Geometry check sheet. Reference: the model listing, model coordinates, mm. A direction names the side the tool comes from. Round coordinates to 2 decimals unless told otherwise and drop trailing zeros. Write each loop counter-clockwise with the first axis right and the second up, starting at its lowest first coordinate (ties: lowest second). Pieces come first, ordered by that corner, then holes. Notation, with made-up numbers: (-5, -31) -> (10, -31) arc R5 ccw to (10, -24) -> close; hole circle Ø5 at (69.25, -15). An arc over 180 degrees is marked (long way). Use a Markdown table: item, result.
```python
from build123d import *

# Parameters (mm, degrees)
BOSS_EXTRUDE1_DEPTH = 4
SKETCH2_R           = 20
BOSS_EXTRUDE2_DEPTH = 4
SKETCH3_R           = 20
BOSS_EXTRUDE3_DEPTH = 4
CUT_EXTRUDE2_DEPTH  = 8
FILLET1_R           = 3
FILLET2_R           = 1


with BuildPart() as part:
    # Sketch1 → Boss-Extrude1 (new, symmetric)
    with BuildSketch(Plane.XY):
        with BuildLine():
            Line((195, 89.5), (-195, 89.5))
            ThreePointArc((-195, 89.5), (-216.213203436, 80.713203436), (-225, 59.5))
            Line((-225, 59.5), (-225, -59.5))
            ThreePointArc((-225, -59.5), (-216.213203436, -80.713203436), (-195, -89.5))
            Line((-195, -89.5), (195, -89.5))
            ThreePointArc((195, -89.5), (216.213203436, -80.713203436), (225, -59.5))
            Line((225, -59.5), (225, 59.5))
            ThreePointArc((225, 59.5), (216.213203436, 80.713203436), (195, 89.5))
        make_face()
    extrude(amount=BOSS_EXTRUDE1_DEPTH, both=True)

    # Sketch2 → Boss-Extrude2 (add, symmetric)
    with BuildSketch(Plane.XY.offset(4)):
        with Locations(Location((-185, 0, 0), (0, 0, 180))):
            Circle(SKETCH2_R)
        with Locations(Location((185, 0, 0), (0, 0, 180))):
            Circle(SKETCH2_R)
    extrude(amount=BOSS_EXTRUDE2_DEPTH, both=True)

    # Sketch3 → Boss-Extrude3 (add, symmetric)
    with BuildSketch(Plane.XY.offset(4)):
        with Locations(Location((0, 0, 0), (0, 0, 180))):
            Circle(SKETCH3_R)
    extrude(amount=BOSS_EXTRUDE3_DEPTH, both=True)

    # Sketch4 → Cut-Extrude2 (cut)
    with BuildSketch(Plane.XY.offset(4)):
        with BuildLine():
            Line((-168.5, 59), (-131.5, 59))
            ThreePointArc((-131.5, 59), (-127.5, 55), (-131.5, 51))
            Line((-131.5, 51), (-168.5, 51))
            ThreePointArc((-168.5, 51), (-172.5, 55), (-168.5, 59))
        make_face()
        with BuildLine():
            Line((168.5, 59), (131.5, 59))
            ThreePointArc((131.5, 59), (127.5, 55), (131.5, 51))
            Line((131.5, 51), (168.5, 51))
            ThreePointArc((168.5, 51), (172.5, 55), (168.5, 59))
        make_face()
        with BuildLine():
            Line((-168.5, -59), (-131.5, -59))
            ThreePointArc((-131.5, -59), (-127.5, -55), (-131.5, -51))
            Line((-131.5, -51), (-168.5, -51))
            ThreePointArc((-168.5, -51), (-172.5, -55), (-168.5, -59))
        make_face()
        with BuildLine():
            Line((168.5, -59), (131.5, -59))
            ThreePointArc((131.5, -59), (127.5, -55), (131.5, -51))
            Line((131.5, -51), (168.5, -51))
            ThreePointArc((168.5, -51), (172.5, -55), (168.5, -59))
        make_face()
    extrude(amount=-CUT_EXTRUDE2_DEPTH, mode=Mode.SUBTRACT)

    # Fillet1
    fillet1_edges = [part.edges().sort_by_distance(p)[0] for p in [
        (225, 0, -4),
        (216.213203436, -80.713203436, -4),
        (0, -89.5, -4),
        (-216.213203436, -80.713203436, -4),
        (216.213203436, -80.713203436, 4),
        (225, 0, 4),
        (216.213203436, 80.713203436, 4),
        (0, 89.5, 4),
        (-216.213203436, 80.713203436, 4),
        (-225, 0, 4),
        (-216.213203436, -80.713203436, 4),
        (-225, 0, -4),
        (0, -89.5, 4),
        (-216.213203436, 80.713203436, -4),
        (0, 89.5, -4),
        (216.213203436, 80.713203436, -4),
    ]]
    fillet(fillet1_edges, radius=FILLET1_R)

    # Fillet2
    fillet2_edges = [part.edges().sort_by_distance(p)[0] for p in [
        (205, 0, 8),
        (-165, 0, 8),
        (20, 0, 8),
    ]]
    fillet(fillet2_edges, radius=FILLET2_R)


solid = part.part
```
(1) Gauge pin test, flat ends, axial feed: pin 1 Ø6 at (y, z) = (40, 1.5) entering from -X; pin 2 Ø3 at (y, z) = (-44.5, 3) entering from +X; pin 3 Ø5 at (y, z) = (-44, 5.5) entering from -X. Record the tip position at first contact, or that the pin passes through.
A:
| item | result |
|---|---|
| pin 1 | stops at x = -225 |
| pin 2 | stops at x = 224.96 |
| pin 3 | stops at x = -224.24 |
(2) Release check for a two-part mould opening along Y. For faces 4 (the face through (216.445, 80.479, 0.014)), 5 (the face through (-150, -59, 0)), 6 (the face through (172.5, 54.9, 0.1)), 7 (the face through (-216.445, -80.479, 0.014)) record: +Y half, -Y half, draft (parallel to the pull), parting line (faces both ways), or undercut.
A:
| item | result |
|---|---|
| face 4 | +Y half |
| face 5 | undercut |
| face 6 | undercut |
| face 7 | -Y half |
(3) Section check A-A on y = -55. Record the cut outline in (x, z).
A:
| item | result |
|---|---|
| outline | (-225, -1) arc R3 ccw to (-222, -4) -> (-172.5, -4) -> (-172.5, 4) -> (-222, 4) arc R3 ccw to (-225, 1) -> close; (-127.5, -4) -> (127.5, -4) -> (127.5, 4) -> (-127.5, 4) -> close; (172.5, -4) -> (222, -4) arc R3 ccw to (225, -1) -> (225, 1) arc R3 ccw to (222, 4) -> (172.5, 4) -> close |
(4) Thickness scan on line 1 (Y direction, x = -142, z = 0.75); line 2 (X direction, y = 54.5, z = -1.25); line 3 (Y direction, x = 119, z = -1.75). Record the ranges inside material, lowest first.
A:
| item | result |
|---|---|
| line 1 | y = -89.5 to -59, -51 to 51, 59 to 89.5 |
| line 2 | x = -224.99 to -172.47, -127.53 to 127.53, 172.47 to 224.99 |
| line 3 | y = -89.4 to 89.4 |
(5) Section check D-D on x = 0. Record the cut outline in (y, z), plus the area to 3 significant figures.
A:
| item | result |
|---|---|
| outline | (-89.5, -1) arc R3 ccw to (-86.5, -4) -> (86.5, -4) arc R3 ccw to (89.5, -1) -> (89.5, 1) arc R3 ccw to (86.5, 4) -> (20, 4) -> (20, 7) arc R1 ccw to (19, 8) -> (-19, 8) arc R1 ccw to (-20, 7) -> (-20, 4) -> (-86.5, 4) arc R3 ccw to (-89.5, 1) -> close |
| area | 1,580 mm2 |
(6) Access from +Z, -Z, +X, -X, +Y, -Y to the whole of each face (thin tool, end or side, straight path). Record for faces 1 (the face through (-3, 20, 4)), 2 (the face through (-3, 1, -4)), 3 (the face through (-172.5, 54.9, 0.1)).
A:
| item | result |
|---|---|
| face 1 | +Z |
| face 2 | -Z, +X, -X, +Y, -Y |
| face 3 | +Z, -Z |
(7) Section check C-C on y = 0. Record the cut outline in (x, z), plus the area to 3 significant figures.
A:
| item | result |
|---|---|
| outline | (-225, -1) arc R3 ccw to (-222, -4) -> (222, -4) arc R3 ccw to (225, -1) -> (225, 1) arc R3 ccw to (222, 4) -> (205, 4) -> (205, 7) arc R1 ccw to (204, 8) -> (166, 8) arc R1 ccw to (165, 7) -> (165, 4) -> (20, 4) -> (20, 7) arc R1 ccw to (19, 8) -> (-19, 8) arc R1 ccw to (-20, 7) -> (-20, 4) -> (-165, 4) -> (-165, 7) arc R1 ccw to (-166, 8) -> (-204, 8) arc R1 ccw to (-205, 7) -> (-205, 4) -> (-222, 4) arc R3 ccw to (-225, 1) -> close |
| area | 4,070 mm2 |
(8) Section check B-B on x = 145. Record the cut outline in (y, z), plus the area to 3 significant figures.
A:
| item | result |
|---|---|
| outline | (-89.5, -1) arc R3 ccw to (-86.5, -4) -> (-59, -4) -> (-59, 4) -> (-86.5, 4) arc R3 ccw to (-89.5, 1) -> close; (-51, -4) -> (51, -4) -> (51, 4) -> (-51, 4) -> close; (59, -4) -> (86.5, -4) arc R3 ccw to (89.5, -1) -> (89.5, 1) arc R3 ccw to (86.5, 4) -> (59, 4) -> close |
| area | 1,300 mm2 |
